Autodesk Inventor part; units mm, degrees
ref_plane "YZ Plane" through (0, 0, 0) normal (1, 0, 0) x (0, 1, 0)
ref_plane "XZ Plane" through (0, 0, 0) normal (0, 1, 0) x (-1, 0, 0)
ref_plane "XY Plane" through (0, 0, 0) normal (0, 0, 1) x (1, 0, 0)
sketch "Szkic1" plane through (0, 0, 0) normal (0, 0, 1) x (1, 0, 0)
  line L0 (-12.5, -10) -> (12.5, -10)
  line L1 (12.5, -10) -> (12.5, 10)
  line L2 (12.5, 10) -> (-12.5, 10)
  line L3 (-12.5, 10) -> (-12.5, -10)
  line L4 (-12.5, -10) -> (12.5, 10) construction
  line L5 (12.5, -10) -> (-12.5, 10) construction
  line L6 (-12.5, 10) -> (16.5, 10)
  line L7 (16.5, 10) -> (16.5, -14)
  line L8 (16.5, -14) -> (-12.5, -14)
  line L9 (-12.5, -14) -> (-12.5, 10)
  point P0 (0, 0)
  dimension "d0" = 25
  dimension "d1" = 20
  dimension "d2" = 4
  dimension "d3" = 4
extrude "Wyciągnięcie proste1" add sketch "Szkic1" against normal blind 9
extrude "Wyciągnięcie proste2" add sketch "Szkic1" along normal blind 10 contours L3 L2 L1 L0
sketch "Szkic2" plane through (0, 0, 10) normal (0, 0, 1) x (1, 0, 0)
  point P0 (0, 0)
  point P1 (0, 0)
sketch "Szkic3" plane through (-12.5, -10, 0) normal (0, -1, 0) x (1, 0, 0)
  line L0 (25, 0) -> (0, 0)
  line L1 (25, 0) -> (25, 10)
  point P0 (12.5, 0)
  point P1 (20, 4)
  dimension "d8" = 5
  dimension "d9" = 4
hole "Otwór1" at (7.5, -10, 4) direction (0, 1, 0) diameter 3.5 end through all
hole "Otwór2" at (0, 0, 10) direction (0, 0, -1) diameter 4 end through all
chamfer "Faza1" distance 2 angle 45 1 edges at (0, 2, 10)
properties part number "table_mount"
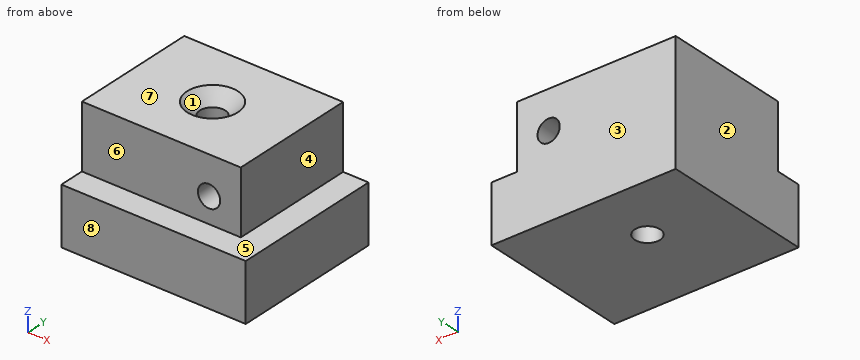
Check sheet for the modelled part. Datum: model origin and axes. Units: mm. Face numbers are marked on the shaded views. A direction names the side the tool comes from. Round coordinates to 2 decimals unless told otherwise and drop trailing zeros. Write each loop counter-clockwise with the first axis right and the second up, starting at its lowest first coordinate (ties: lowest second). Pieces come first, ordered by that corner, then holes. Notation, with made-up numbers: (-22.75, -2) -> (-13.75, -2) arc R15 ccw to (-13.75, 9) -> close; hole circle Ø5 at (-32.75, 15.25). An arc over 180 degrees is marked (long way). Put each result on its own line as item: value.
(1) Tool access check on the marked faces 4, 5, 6, 7 and 8. Record the directions out of +Z, -Z, +X, -X, +Y, -Y that give a thin tool (end or side, any length) a straight path to the whole face; none if there is none.
Values found:
face 4: +Z, +X, +Y, -Y
face 5: +Z, +X, -Y
face 6: +Z, +X, -X, -Y
face 7: +Z, +X, -X, +Y, -Y
face 8: +Z, -Z, +X, -X, -Y
(2) Mould release check, pull along Y, two halves, no side actions. Record for the marked faces 1, 2 and 3: released by +Y, released by -Y, zero draft, split by the parting line, or undercut.
Values found:
face 1: undercut
face 2: zero draft
face 3: released by +Y
(3) Sectioned sample at A-A (y = 0). Enter the section's corners in (x, z).
Values found:
outline: (-12.5, -9) -> (-2, -9) -> (-2, 8) -> (-4, 10) -> (-12.5, 10) -> close; (2, -9) -> (16.5, -9) -> (16.5, 0) -> (12.5, 0) -> (12.5, 10) -> (4, 10) -> (2, 8) -> close; hole circle Ø3.5 at (7.5, 4)
(4) Material ranges on line 1 (Z direction, x = 7.5, y = -4.5); line 2 (Y direction, x = 0, z = -1.25); line 3 (X direction, y = -5, z = 4), recorded low to high.
Values found:
line 1: z = -9 to 2.25, 5.75 to 10
line 2: y = -14 to -2, 2 to 10
line 3: x = -12.5 to 5.75, 9.25 to 12.5
(5) Sectioned sample at C-C (z = 4). Enter the section's corners in (x, y).
Values found:
outline: (-12.5, -10) -> (5.75, -10) -> (5.75, 10) -> (-12.5, 10) -> close; (9.25, -10) -> (12.5, -10) -> (12.5, 10) -> (9.25, 10) -> close; hole circle Ø4 at (0, 0)
(6) Go/stop test with flat-tipped pins: pin 1 Ø3 at (x, z) = (1, 4) entering from -Y; pin 2 Ø4.5 at (x, y) = (0, 0) entering from +Z; pin 3 Ø3 at (x, y) = (1, 0) entering from +Z. Record where each tip stops, or that it passes through.
Values found:
pin 1: stops at y = -10
pin 2: stops at z = 8.25
pin 3: stops at z = 8.5
(7) Sectioned sample at D-D (y = -5). Enter the section's corners in (x, z).
Values found:
outline: (-12.5, -9) -> (16.5, -9) -> (16.5, 0) -> (12.5, 0) -> (12.5, 10) -> (-12.5, 10) -> close; hole circle Ø3.5 at (7.5, 4)
(8) Sectioned sample at B-B (x = 7.5). Enter the section's corners in (y, z).
Values found:
outline: (-14, -9) -> (10, -9) -> (10, 2.25) -> (-10, 2.25) -> (-10, 0) -> (-14, 0) -> close; (-10, 5.75) -> (10, 5.75) -> (10, 10) -> (-10, 10) -> close
